Geometry: final body of the model. Coordinates: model frame, mm. Face numbers are marked on the shaded views. Give positions to 0.01 mm unless a question says otherwise; leave off trailing zeros. Write each loop counter-clockwise with the first axis right and the second up, starting at its lowest first coordinate (ties: lowest second). Pieces come first, ordered by that corner, then holes. Notation, with made-up numbers: (19.25, 9.5) -> (58.25, 9.5) arc R6 cw to (58.25, 19.5) -> close; hole circle Ø3 at (36, 65.25). An arc over 180 degrees is marked (long way). Answer as a JSON object with one key per item and string values. Group by question number.
(1) Material intervals for probe 1 along Y at (x, z) = (-6, -4.4); probe 2 along Y at (x, z) = (9, -1.75); probe 3 along Z at (x, y) = (-30, 9), sorted ascending.
(2) Contact query for flat-ended pins moving along their axis: pin 1 Ø2.5 at (x, y) = (0, 55.75) entering from +Z; pin 2 Ø3 at (x, y) = (-15.5, -42) entering from -Z; pin 3 Ø0.8 at (y, z) = (13.5, -4.5) entering from -X; pin 4 Ø0.9 at (x, y) = (29.98, -20) entering from +Z. Output: stop coordinate, or through.
(3) Draft query along X for the marked faces 1 and 2. Return one class per face: +X half, -X half, draft (parallel to the pull), parting line (faces both ways), or undercut.
(4) Section query A-A on x = -18.5. Output: boundary loops of the cut face in (y, z).
(5) Section query B-B on y = 31. Output: boundary loops of the cut face in (x, z), plus the area to 3 significant figures.
from build123d import *

# Parameters (mm, degrees)
SKETCH1_W           = 82
SKETCH1_H           = 122
BOSS_EXTRUDE1_DEPTH = 4
SKETCH2_W           = 76
SKETCH2_H           = 116
CUT_EXTRUDE1_DEPTH  = 0.0001
SKETCH6_W           = 78
SKETCH6_H           = 118
SKETCH6_W_2         = 76
SKETCH6_H_2         = 116
BOSS_EXTRUDE4_DEPTH = 1
SKETCH3_R           = 2
BOSS_EXTRUDE2_DEPTH = 1
SKETCH5_R           = 0.75
CUT_EXTRUDE2_DEPTH  = 74.66816816
SKETCH7_R           = 0.75
CUT_EXTRUDE3_DEPTH  = 74.607059444


with BuildPart() as part:
    # Sketch1 → Boss-Extrude1 (new body)
    with BuildSketch(Plane.XY):
        Rectangle(SKETCH1_W, SKETCH1_H)
    extrude(amount=-BOSS_EXTRUDE1_DEPTH)

    # Sketch2 → Cut-Extrude1 (cut)
    with BuildSketch(Plane(origin=(0, 0, -4), x_dir=(-1, 0, 0), z_dir=(0, 0, -1))):
        Rectangle(SKETCH2_W, SKETCH2_H)
    extrude(amount=-CUT_EXTRUDE1_DEPTH, mode=Mode.SUBTRACT)

    # Sketch6 → Boss-Extrude4 (add)
    with BuildSketch(Plane(origin=(0, 0, -4), x_dir=(-1, 0, 0), z_dir=(0, 0, -1))):
        Rectangle(SKETCH6_W, SKETCH6_H)
        Rectangle(SKETCH6_W_2, SKETCH6_H_2, mode=Mode.SUBTRACT)
    extrude(amount=BOSS_EXTRUDE4_DEPTH)

    # Sketch3 → Boss-Extrude2 (add)
    with BuildSketch(Plane(origin=(0, 0, -3.9999), x_dir=(-1, 0, 0), z_dir=(0, 0, -1))):
        with Locations(Location((30, 50, 0), (0, 0, 180))):
            Circle(SKETCH3_R)
        with Locations(Location((-30, 50, 0), (0, 0, 180))):
            Circle(SKETCH3_R)
        with Locations(Location((30, -20, 0), (0, 0, 180))):
            Circle(SKETCH3_R)
        with Locations(Location((-30, -20, 0), (0, 0, 180))):
            Circle(SKETCH3_R)
    extrude(amount=BOSS_EXTRUDE2_DEPTH)

    # Sketch5 → Cut-Extrude2 (cut, through all)
    with BuildSketch(Plane(origin=(0, 0, -4.9999), x_dir=(-1, 0, 0), z_dir=(0, 0, -1))):
        with Locations((-30, 50)):
            Circle(SKETCH5_R)
        with Locations((29.999997646, 50.016807976)):
            Circle(SKETCH5_R)
        with Locations((30.019606951, -19.983189277)):
            Circle(SKETCH5_R)
        with Locations((-29.980390695, -19.999997253)):
            Circle(SKETCH5_R)
    extrude(amount=-CUT_EXTRUDE2_DEPTH, mode=Mode.SUBTRACT)

    # Sketch7 → Cut-Extrude3 (cut, through all)
    with BuildSketch(Plane(origin=(0, 0, -3.9999), x_dir=(-1, 0, 0), z_dir=(0, 0, -1))):
        with Locations((13.5, 57.25)):
            Circle(SKETCH7_R)
        with Locations((10.5, 57.25)):
            Circle(SKETCH7_R)
        with Locations((7.5, 57.25)):
            Circle(SKETCH7_R)
        with Locations((4.5, 57.25)):
            Circle(SKETCH7_R)
        with Locations((1.5, 57.25)):
            Circle(SKETCH7_R)
        with Locations((-1.5, 57.25)):
            Circle(SKETCH7_R)
        with Locations((-4.5, 57.25)):
            Circle(SKETCH7_R)
        with Locations((-7.5, 57.25)):
            Circle(SKETCH7_R)
        with Locations((-10.5, 57.25)):
            Circle(SKETCH7_R)
        with Locations((-13.5, 57.25)):
            Circle(SKETCH7_R)
        with Locations((12, 55.75)):
            Circle(SKETCH7_R)
        with Locations((9, 55.75)):
            Circle(SKETCH7_R)
        with Locations((6, 55.75)):
            Circle(SKETCH7_R)
        with Locations((3, 55.75)):
            Circle(SKETCH7_R)
        with Locations((0, 55.75)):
            Circle(SKETCH7_R)
        with Locations((-3, 55.75)):
            Circle(SKETCH7_R)
        with Locations((-6, 55.75)):
            Circle(SKETCH7_R)
        with Locations((-9, 55.75)):
            Circle(SKETCH7_R)
        with Locations((-12, 55.75)):
            Circle(SKETCH7_R)
    extrude(amount=-CUT_EXTRUDE3_DEPTH, mode=Mode.SUBTRACT)


solid = part.part
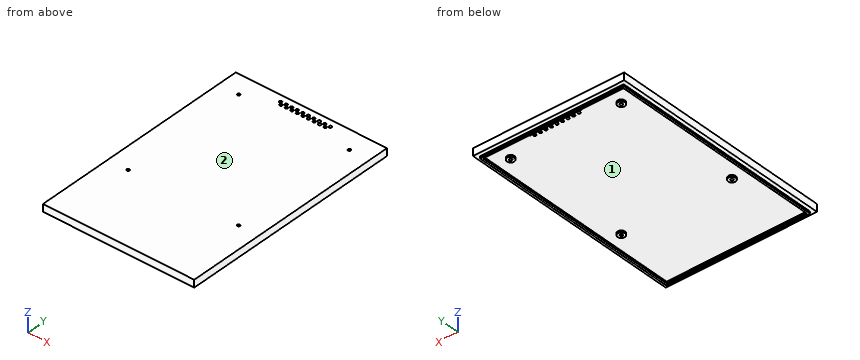
Answer list:
{
 "1": {"probe 1": "-59 to -58, 58 to 59", "probe 2": "-61 to 55, 56.5 to 61", "probe 3": "-4 to 0"},
 "2": {"pin 1": "z = 0", "pin 2": "z = -4", "pin 3": "x = -39", "pin 4": "through"},
 "3": {"face 1": "undercut", "face 2": "draft"},
 "4": {"outline": "(-61, -4) -> (-59, -4) -> (-59, -5) -> (-58, -5) -> (-58, -4) -> (58, -4) -> (58, -5) -> (59, -5) -> (59, -4) -> (61, -4) -> (61, 0) -> (-61, 0) -> close"},
 "5": {"outline": "(-41, -4) -> (-39, -4) -> (-39, -5) -> (-38, -5) -> (-38, -4) -> (38, -4) -> (38, -5) -> (39, -5) -> (39, -4) -> (41, -4) -> (41, 0) -> (-41, 0) -> close", "area": "330 mm2"}
}
